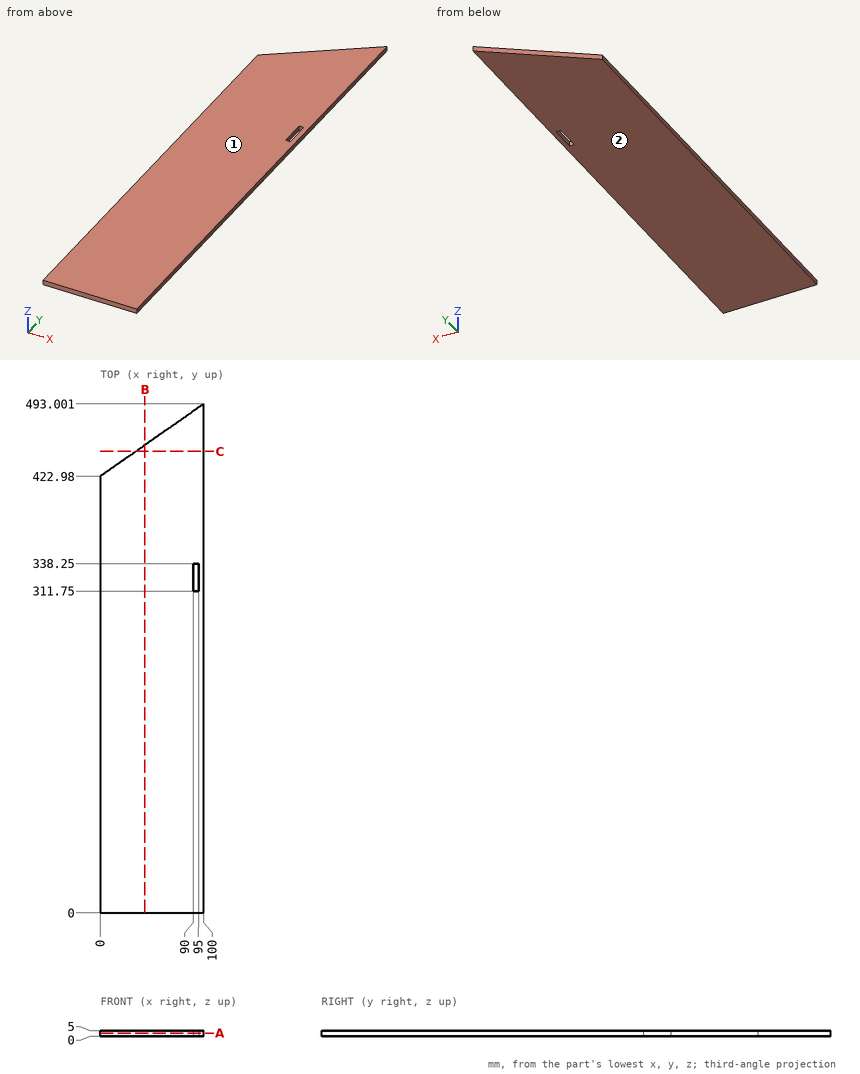
Answer from the drawing. Dimensions are ordinates in mm from the lowest x, y and z of the part. Round coordinates to 2 decimals unless told otherwise and drop trailing zeros. Loops run counter-clockwise (first coordinate to the right, second up) from the corner with the lowest first, then second, coordinate; pieces in that order, holes last.
1) A cutting plane is placed at A-A on z = 2.7. Determine the outline of the cut face in (x, y).
Outcome:
outline: (0, 0) - (100, 0) - (100, 493) - (0, 422.98) - close; hole (90, 311.75) - (95, 311.75) - (95, 338.25) - (90, 338.25) - close
2) A cutting plane is placed at C-C on y = 447. Determine the outline of the cut face in (x, z).
Outcome:
outline: (34.3, 0) - (100, 0) - (100, 5) - (34.3, 5) - close
3) Consider line 1 (Y direction, x = 92, z = 3.1); line 2 (Y direction, x = 79, z = 3.45); line 3 (Y direction, x = 78, z = 1.75) (1 decimal). Determine where each line is inside the solid, lowest interval first.
Outcome:
line 1: y = 0 to 311.75, 338.25 to 487.4
line 2: y = 0 to 478.3
line 3: y = 0 to 477.6
4) For a pull along Z with two mould halves and no side action, classify the marked faces 1 and 2 as released by +Z, released by -Z, zero draft, split by the parting line, or undercut.
Outcome:
face 1: released by +Z
face 2: released by -Z
5) A cutting plane is placed at B-B on x = 43. Determine the outline of the cut face in (y, z).
Outcome:
outline: (0, 0) - (453.09, 0) - (453.09, 5) - (0, 5) - close
6) Given P1, Ø2.5, axis at x = 92, z = 3, coming from the +Y side (1 decimal), flat-ended and moving along its own axis, determine where the tip first touches the part or whether it passes through.
Outcome:
P1: stops at y = 488.3
